```python
from build123d import *

# Parameters (mm, degrees)
F0_R      = 15.628254
F1_DEPTH  = 7.62
F2_R      = 12.192
F3_DEPTH  = 25.4
F3_FACE_R = 12.192
F4_DEPTH  = 23.368
F5_R      = 0.508
F6_DEPTH  = 12.7


with BuildPart() as f1:
    # F0 (on Top) → F1 (new body)
    with BuildSketch(Plane.XY):
        with Locations((-47.424259, 29.709655)):
            Circle(F0_R)
    extrude(amount=F1_DEPTH)

    # F2 (on Top) → F3 (join)
    with BuildSketch(Plane.XY):
        with Locations((-47.505132, 29.709655)):
            Circle(F2_R)
    extrude(amount=F3_DEPTH)

    # F3_face (on face) → F4 (cut, symmetric)
    with BuildSketch(Plane(origin=(-47.505132, 29.709655, 25.4), x_dir=(1, 0, 0), z_dir=(0, 0, 1))):
        Circle(F3_FACE_R)
    extrude(amount=F4_DEPTH, both=True, mode=Mode.SUBTRACT)

    # F5 (on Top) → F6 (cut, symmetric)
    with BuildSketch(Plane.XY):
        with Locations((-47.353999, 29.709655)):
            Circle(F5_R)
    extrude(amount=F6_DEPTH, both=True, mode=Mode.SUBTRACT)


solid = f1.part
```
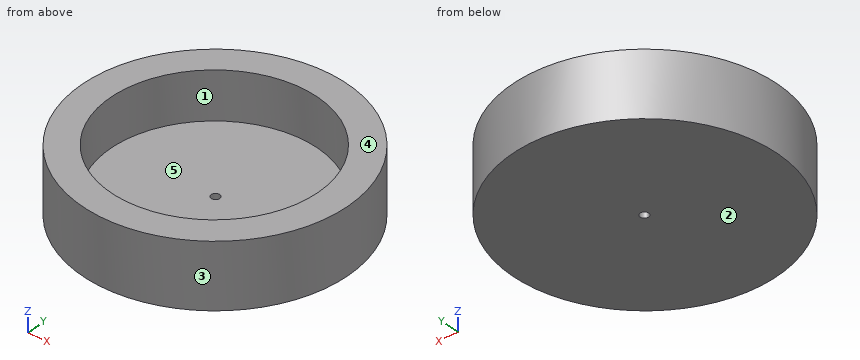
Geometry check sheet. Reference: the model listing, model coordinates, mm. Face numbers are marked on the shaded views. A direction names the side the tool comes from. Give positions to 0.01 mm unless a question says otherwise; leave off trailing zeros. Write each loop counter-clockwise with the first axis right and the second up, starting at its lowest first coordinate (ties: lowest second). Pieces come first, ordered by that corner, then holes.
1) Access from +Z, -Z, +X, -X, +Y, -Y to the whole of each face (thin tool, end or side, straight path). Record for the marked faces 1 and 2.
2) Section check D-D, the plane y = 43. Record the boundary of the cut face in (x, z), and give its area (3 significant figures).
3) Section check A-A, the plane x = -54. Record the boundary of the cut face in (y, z).
4) Section check B-B, the plane y = 26. Record the boundary of the cut face in (x, z).
5) Release check for a two-part mould opening along Y. For the marked faces 3, 4 and 5 record: pulls with the +Y half, pulls with the -Y half, needs draft (parallel to the pull), parting line crosses it, or undercut.
6) Gauge pin test, flat end, axial feed: pin 1 (1.2 mm diameter, centred on x = -47.35, y = 29.71, fed in from +Z). Record the tip position at first contact, or that the pin passes through.
7) Section check C-C, the plane z = 0.75. Record the boundary of the cut face in (x, y).
8) Material ranges on L1, parallel to Y at x = -55.5, z = 4.75; L2, parallel to Y at x = -51, z = 6.5; L3, parallel to Z at x = -46, y = 21, recorded low to high.
Computed:
1. face 1: +Z
1. face 2: -Z, +X, -X, +Y, -Y
2. outline: (-55.65, 0) - (-39.2, 0) - (-39.2, 7.62) - (-55.65, 7.62) - close
2. area: 125 mm2
3. outline: (15.53, 0) - (43.89, 0) - (43.89, 7.62) - (40.03, 7.62) - (40.03, 2.03) - (19.39, 2.03) - (19.39, 7.62) - (15.53, 7.62) - close
4. outline: (-62.61, 0) - (-32.24, 0) - (-32.24, 7.62) - (-35.89, 7.62) - (-35.89, 2.03) - (-59.12, 2.03) - (-59.12, 7.62) - (-62.61, 7.62) - close
5. face 3: parting line crosses it
5. face 4: needs draft
5. face 5: undercut
6. pin 1: stops at z = 2.03
7. outline: circle Ø31.26 at (-47.42, 29.71); hole circle Ø1.02 at (-47.35, 29.71)
8. L1: y = 16.33 to 20.5, 38.91 to 43.09
8. L2: y = 14.5 to 18.03, 41.39 to 44.92
8. L3: z = 0 to 2.03
